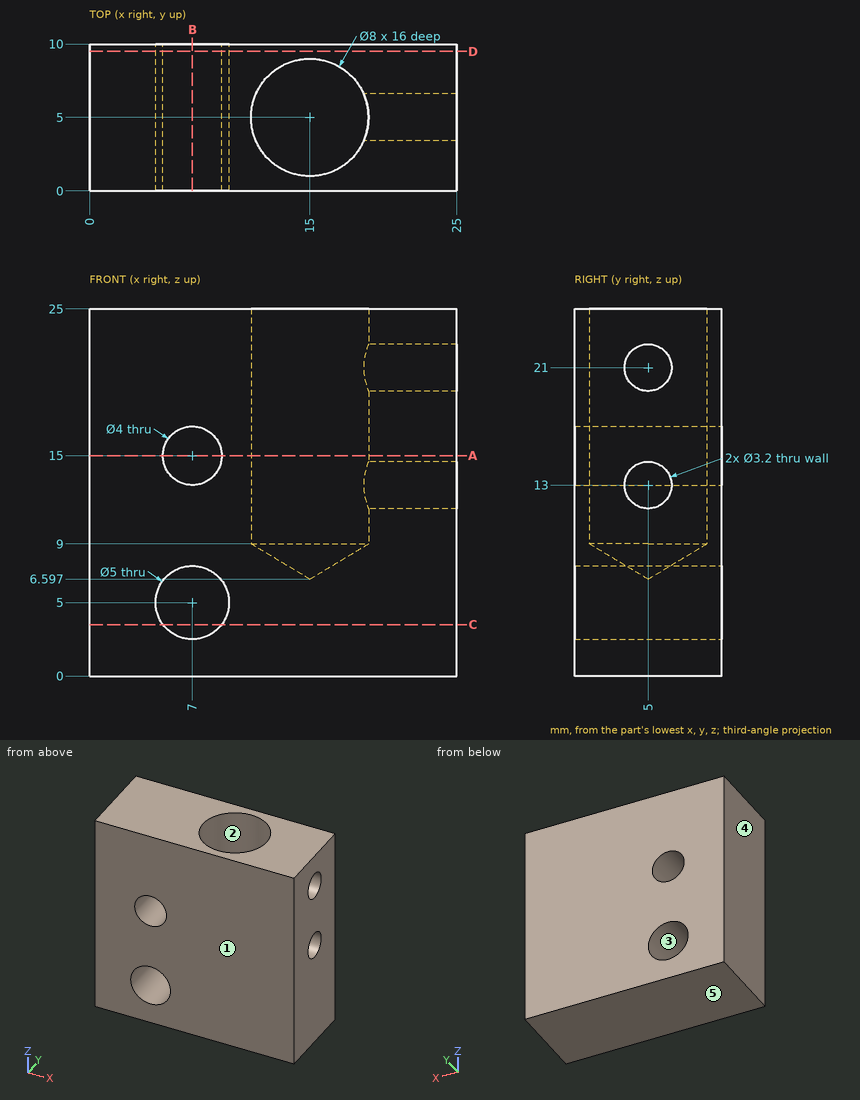
Geometry: see drawing. Coordinates: mm, zero at the bounding-box minimum. A direction names the side the tool comes from. Round coordinates to 2 decimals unless told otherwise and drop trailing zeros. Write each loop counter-clockwise with the first axis right and the second up, starting at its lowest first coordinate (ties: lowest second). Pieces come first, ordered by that corner, then holes. Notation, with made-up numbers: M 52.25,48.5 L 86.25,48.5 A22 ccw 86.25,68.5 Z; hole C 33.5,40.5 d7. An arc over 180 degrees is marked long. Answer in a Markdown table with one row per item. Add a question column.
(1) Cut plane B-B, the plane x = 7. Return the cut outline in (y, z), then the cut area to 3 significant figures.
(2) Contact query for a flat-ended pin moving along its axis: pin 1 (2.5 mm diameter, centred on y = 5, z = 13, fed in from +X). Output: stop coordinate, or through.
(3) Cut plane A-A, the plane z = 15. Return the cut outline in (x, y).
(4) Draft query along X for the marked faces 3, 4 and 5. Return one class per face: pulls with the +X half, pulls with the -X half, needs draft (parallel to the pull), parting line crosses it, or undercut.
(5) Cut plane D-D, the plane y = 9.5. Return the cut outline in (x, z), then the cut area to 3 significant figures.
(6) Cut plane C-C, the plane z = 3.5. Return the cut outline in (x, y).
(7) Ray query, L1, parallel to Z at x = 22, y = 5; L2, parallel to Z at x = 7, y = 4.25; L3, parallel to Y at x = 20.5, z = 13. Return the intervals inside material, ascending.
(8) Reachability of the marked faces 1 and 2 from +Z, -Z, +X, -X, +Y, -Y: full face, straight path, thin tool, end or side. Return the list, or none.
Established:
| question | item | result |
|---|---|---|
| 1 | outline | M 0,0 L 10,0 L 10,2.5 L 0,2.5 Z; M 0,7.5 L 10,7.5 L 10,13 L 0,13 Z; M 0,17 L 10,17 L 10,25 L 0,25 Z |
| 1 | area | 160 mm² |
| 2 | pin 1 | x = 11.2 |
| 3 | outline | M 0,0 L 5,0 L 5,10 L 0,10 Z; M 9,0 L 25,0 L 25,10 L 9,10 Z; hole C 15,5 d8 |
| 4 | face 3 | undercut |
| 4 | face 4 | pulls with the -X half |
| 4 | face 5 | needs draft |
| 5 | outline | M 0,0 L 25,0 L 25,25 L 0,25 Z; hole C 7,5 d5; hole C 7,15 d4 |
| 5 | area | 593 mm² |
| 6 | outline | M 0,0 L 5,0 L 5,10 L 0,10 Z; M 9,0 L 25,0 L 25,10 L 9,10 Z |
| 7 | L1 | 0 to 11.4, 14.6 to 19.4, 22.6 to 25 |
| 7 | L2 | 0 to 2.5, 7.5 to 13, 17 to 25 |
| 7 | L3 | 0 to 3.4, 6.6 to 10 |
| 8 | face 1 | +Z, -Z, +X, -X, -Y |
| 8 | face 2 | +Z |
